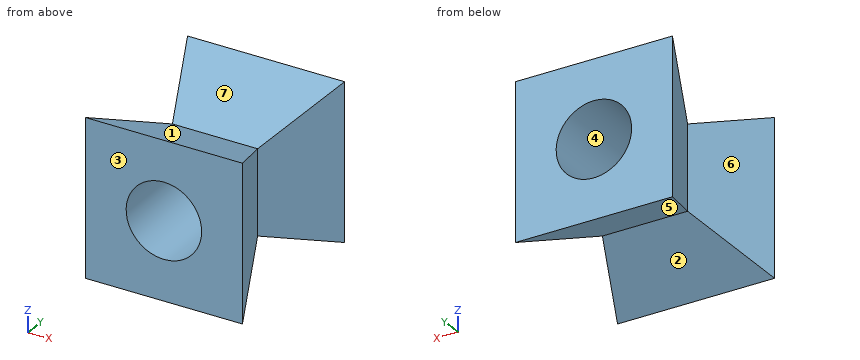
```python
from build123d import *

# Parameters (mm, degrees)
BOSS_EXTRU_2_DEPTH           = 52
ESQUISSE3_R                  = 25
ENL_V_MAT_EXTRU_1_DEPTH      = 134.985073796
ENL_V_MAT_EXTRU_2_DEPTH      = 93.433760066
ENL_V_MAT_EXTRU_2_DEPTH_BACK = 93.433760066


with BuildPart() as part:
    # Esquisse2 → Boss.-Extru.2 (new, symmetric)
    with BuildSketch(Plane.XY):
        Polygon((28.229410292, 0), (52, -56), (-52, -56), (-28.229410292, 0), align=None)
        Polygon((-28.229410292, 0), (-52, 56), (52, 56), (28.229410292, 0), align=None)
    extrude(amount=BOSS_EXTRU_2_DEPTH, both=True)

    # Esquisse3 → Enlèv. mat.-Extru.1 (cut, through all)
    with BuildSketch(Plane(origin=(0, 56, 0), x_dir=(1, 0, 0), z_dir=(0, 1, 0))):
        with Locations(Location((0, 0, 0), (0, 0, 270))):
            Circle(ESQUISSE3_R)
    extrude(amount=-ENL_V_MAT_EXTRU_1_DEPTH, mode=Mode.SUBTRACT)

    # Esquisse4 → Enlèv. mat.-Extru.2 (cut, two sides: drawn at the far end of the back side and taken through both)
    with BuildSketch(Plane(origin=(0, 0, 0), x_dir=(0, 0, -1), z_dir=(1, 0, 0)).offset(-ENL_V_MAT_EXTRU_2_DEPTH_BACK)):
        Polygon((-28.229410292, 0), (-52, 56), (-52, 1.282618983), (-52, -56), align=None)
        Polygon((52, 56), (28.229410292, 0), (52, -56), align=None)
    extrude(amount=ENL_V_MAT_EXTRU_2_DEPTH + ENL_V_MAT_EXTRU_2_DEPTH_BACK, mode=Mode.SUBTRACT)


solid = part.part
```
Geometry: final body of the model. Coordinates: model frame, mm. Face numbers are marked on the shaded views. A direction names the side the tool comes from. Round coordinates to 2 decimals unless told otherwise and drop trailing zeros. Loops run counter-clockwise (first coordinate to the right, second up) from the corner with the lowest first, then second, coordinate; pieces in that order, holes last. Notation, with made-up numbers: (41.5, 68.5) -> (70.5, 68.5) arc R17 ccw to (70.5, 74.5) -> close; hole circle Ø11 at (63, -9.75). An arc over 180 degrees is marked (long way). Use one line per item in the form item = value. Start each with the question number.
1) Section C-C on y = 22. Output: boundary loops of the cut face in (x, z).
2) Access query for the marked faces 5, 6 and 7. Directions: +Z, -Z, +X, -X, +Y, -Y. A direction counts if a zero-diameter tool reaches every point of the face in a straight line with its end or side. Return the directions, or none.
3) Line query: L1, parallel to X at y = 5.5, z = 0; L2, parallel to Y at x = -13, z = 45; L3, parallel to Y at x = -4.5, z = 46.5. Output: solid intervals per line, ascending.
4) Section B-B on x = 40. Output: boundary loops of the cut face in (y, z).
5) Section D-D on z = -16. Output: boundary loops of the cut face in (x, y).
6) Draft query along Z for the marked faces 1, 2, 3 and 4. Return one class per face: released by +Z, released by -Z, zero draft, split by the parting line, or undercut.
7) Section A-A on z = 0. Output: boundary loops of the cut face in (x, y), then the cut area to 3 significant figures.
8) First-contact query: P1, Ø2, axis at y = 37.5, z = 31, coming from the +X side; P2, Ø12, axis at x = -12, z = 13.5, coming from the +Y side; P3, Ø8, axis at y = 11, z = 1, coming from the +X side; P4, Ø10, axis at y = -22, z = 41.5, coming from the -X side. Flat tips, straight axial feed; report the tip coordinate or a pass-through.
Response:
q1.outline = (-37.57, -37.57) -> (37.57, -37.57) -> (37.57, 37.57) -> (-37.57, 37.57) -> close; hole circle Ø50 at (0, 0)
q2.face_5 = -Z, +X, -X
q2.face_6 = +Z, -Z, -X
q2.face_7 = +Z, +X, -X
q3.L1 = -30.56 to -25, 25 to 30.56
q3.L2 = -56 to -39.51, 39.51 to 56
q3.L3 = -56 to -43.04, 43.04 to 56
q4.outline = (-56, -52) -> (-27.73, -40) -> (-27.73, 40) -> (-56, 52) -> close; (27.73, -40) -> (56, -52) -> (56, 52) -> (27.73, 40) -> close
q5.outline = (-52, -56) -> (-19.21, -56) -> (-19.21, 56) -> (-52, 56) -> (-28.23, 0) -> close; (19.21, -56) -> (52, -56) -> (28.23, 0) -> (52, 56) -> (19.21, 56) -> close
q6.face_1 = released by +Z
q6.face_2 = released by -Z
q6.face_3 = zero draft
q6.face_4 = undercut
q7.outline = (-52, -56) -> (-25, -56) -> (-25, 56) -> (-52, 56) -> (-28.23, 0) -> close; (25, -56) -> (52, -56) -> (28.23, 0) -> (52, 56) -> (25, 56) -> close
q7.area = 3,390 mm^2
q8.P1 = 44.57
q8.P2 = through
q8.P3 = 34.6
q8.P4 = -39.52
